```python
from build123d import *

# Parameters (mm, degrees)
BOSS_SWITCH_BODY_DEPTH            = 3
SKETCH1_W                         = 2.994375291
SKETCH1_H                         = 2.409101515
SKETCH1_W_2                       = 3.994375291
SKETCH1_H_2                       = 3.957767538
BOSS_FLANGE_WIDTH_DEPTH           = 5
BOSS_FLANGE_HEIGHT_REACH          = 36.354
SKETCH2_W                         = 4
SKETCH2_H                         = 3.957767538
SKETCH2_W_2                       = 8
SKETCH2_H_2                       = 1.451333978
SKETCH17_W                        = 15.1675
SKETCH17_H                        = 4
BOSS_FLANGE_SUPPORT_DEPTH         = 13.053634428
CUT_WALL_GAP_DEPTH                = 1
TAP_DRILL_FOR_M2X0_4_TAP1_D       = 1.6
M2_CLEARANCE_HOLE2_D              = 2.4
M2_CLEARANCE_HOLE2_DEPTH          = 13.462735941
CHAMFER_FLANGE_SUPPORT_3_SIZE     = 1
FILLET1_R                         = 1
FILLET2_R                         = 0.5
SKETCH28_W                        = 5.9675
SKETCH28_H                        = 12.095866891
CUT_PRINT_SUPPORT_CLEARANCE_DEPTH = 33.624103931


with BuildPart() as part:
    # Sketch-SwitchBossUp → Boss-Switch Body (new body)
    with BuildSketch(Plane.XY):
        with BuildLine():
            Line((-5.697895702, 26.949658376), (-5.524247524, 25.964850623))
            ThreePointArc((-5.524247524, 25.964850623), (-6.169751391, 25.553619307), (-6.3354071, 24.806394693))
            Line((-6.3354071, 24.806394693), (-4.07798079, 12.003893904))
            ThreePointArc((-4.07798079, 12.003893904), (-3.666749473, 11.358390037), (-2.919524859, 11.192734328))
            Line((-2.919524859, 11.192734328), (-2.734924291, 10.145812481))
            Line((-2.734924291, 10.145812481), (-1.956559213, 9.844099378))
            Line((-1.956559213, 9.844099378), (-1.327187553, 9.600139722))
            Line((-1.327187553, 9.600139722), (-1.735258621, 8.547390389))
            ThreePointArc((-1.735258621, 8.547390389), (-1.752158006, 8.457034961), (-1.735258621, 8.366679532))
            Line((-1.735258621, 8.366679532), (-1.327187553, 7.313930199))
            Line((-1.327187553, 7.313930199), (-1.956559213, 7.069970543))
            Line((-1.956559213, 7.069970543), (-0.547014535, 3.433600952))
            Line((-0.547014535, 3.433600952), (0.082357125, 3.677560608))
            Line((0.082357125, 3.677560608), (0.805200549, 1.81275569))
            Line((0.805200549, 1.81275569), (-0.12720191, 1.451333978))
            Line((-0.12720191, 1.451333978), (-0.12720191, 0))
            Line((-0.12720191, 0), (2.867173381, 0))
            Line((2.867173381, 0), (2.867173381, 2.409101515))
            Line((2.867173381, 2.409101515), (2.343664607, 2.409101515))
            Line((2.343664607, 2.409101515), (1.411262148, 2.047679803))
            Line((1.411262148, 2.047679803), (0.688418723, 3.912484721))
            Line((0.688418723, 3.912484721), (1.317790383, 4.156444377))
            Line((1.317790383, 4.156444377), (1.063052687, 4.813621425))
            Line((1.063052687, 4.813621425), (3.125189653, 5.612955517))
            Line((3.125189653, 5.612955517), (3.125189653, 6.948407561))
            Line((3.125189653, 6.948407561), (2.225005405, 7.93492645))
            Line((2.225005405, 7.93492645), (0.162983401, 7.13563692))
            Line((0.162983401, 7.13563692), (-0.091754295, 7.792813968))
            Line((-0.091754295, 7.792813968), (-0.721125955, 7.548854312))
            Line((-0.721125955, 7.548854312), (-1.038134762, 8.366679532))
            ThreePointArc((-1.038134762, 8.366679532), (-1.055034148, 8.457034961), (-1.038134762, 8.547390389))
            Line((-1.038134762, 8.547390389), (-0.721125955, 9.365215609))
            Line((-0.721125955, 9.365215609), (-0.091754295, 9.121255953))
            Line((-0.091754295, 9.121255953), (1.317790383, 12.757625544))
            Line((1.317790383, 12.757625544), (0.688418723, 13.0015852))
            Line((0.688418723, 13.0015852), (1.411262148, 14.866390118))
            Line((1.411262148, 14.866390118), (2.343664607, 14.504968406))
            Line((2.343664607, 14.504968406), (2.867173381, 14.504968406))
            Line((2.867173381, 14.504968406), (2.867173381, 18.462735944))
            Line((2.867173381, 18.462735944), (-0.111637615, 18.462735944))
            Line((-0.111637615, 18.462735944), (-1.12720191, 18.462735944))
            Line((-1.12720191, 18.462735944), (-1.12720191, 15.462735944))
            Line((-1.12720191, 15.462735944), (-0.12720191, 15.462735944))
            Line((-0.12720191, 15.462735944), (0.805200549, 15.101314231))
            Line((0.805200549, 15.101314231), (0.082357125, 13.236509313))
            Line((0.082357125, 13.236509313), (-0.547014535, 13.480468969))
            Line((-0.547014535, 13.480468969), (-1.059112089, 12.159350171))
            Line((-1.059112089, 12.159350171), (-2.346896051, 19.462735944))
            Line((-2.346896051, 19.462735944), (3.767173381, 19.462735944))
            Line((3.767173381, 19.462735944), (3.767173381, 25.857619356))
            Line((3.767173381, 25.857619356), (1.767173381, 25.857619356))
            Line((1.767173381, 25.857619356), (1.767173381, 21.462735944))
            Line((1.767173381, 21.462735944), (-2.699550012, 21.462735944))
            Line((-2.699550012, 21.462735944), (-3.728280196, 27.296954732))
            ThreePointArc((-3.728280196, 27.296954732), (-2.874356585, 27.992742953), (-2.319025652, 28.944012807))
            ThreePointArc((-2.319025652, 28.944012807), (-2.76728001, 29.905297381), (-3.728564583, 29.457043022))
            ThreePointArc((-3.728564583, 29.457043022), (-4.944660137, 28.436617692), (-6.436422172, 28.97957467))
            ThreePointArc((-6.436422172, 28.97957467), (-7.493046212, 29.072017295), (-7.585488837, 28.015393255))
            ThreePointArc((-7.585488837, 28.015393255), (-6.738295005, 27.311426358), (-5.697895702, 26.949658376))
        make_face()
    extrude(amount=BOSS_SWITCH_BODY_DEPTH)

    # Sketch1 → Boss-Flange Width (add)
    with BuildSketch(Plane(origin=(0, 0, 0), x_dir=(-1, 0, 0), z_dir=(0, 0, -1))):
        with Locations((-1.369985736, 1.204550758)):
            Rectangle(SKETCH1_W, SKETCH1_H)
        with Locations((-0.869985736, 16.483852175)):
            Rectangle(SKETCH1_W_2, SKETCH1_H_2)
    extrude(amount=BOSS_FLANGE_WIDTH_DEPTH)

    # Boss-Flange Height: up to this face of the body (flat: up to its plane)
    boss_flange_height_end = Plane(part.part.faces().sort_by_distance((-0.12720191, 1.077409098, -1.438016547))[0])
    # Sketch2 → Boss-Flange Height (add, up to the picked face)
    with BuildSketch(Plane(origin=(-12.300326619, 0, 0), x_dir=(0, 0, -1), z_dir=(1, 0, 0)), mode=Mode.PRIVATE) as boss_flange_height_sk1:
        with Locations((3, 16.483852175)):
            Rectangle(SKETCH2_W, SKETCH2_H)
    boss_flange_height_tool1 = split(extrude(boss_flange_height_sk1.sketch, amount=BOSS_FLANGE_HEIGHT_REACH, mode=Mode.PRIVATE), bisect_by=boss_flange_height_end, keep=Keep.BOTH, mode=Mode.PRIVATE)
    # Sketch2 → Boss-Flange Height (add, up to the picked face)
    with BuildSketch(Plane(origin=(-12.300326619, 0, 0), x_dir=(0, 0, -1), z_dir=(1, 0, 0)), mode=Mode.PRIVATE) as boss_flange_height_sk2:
        with Locations((1, 0.725666989)):
            Rectangle(SKETCH2_W_2, SKETCH2_H_2)
    boss_flange_height_tool2 = split(extrude(boss_flange_height_sk2.sketch, amount=BOSS_FLANGE_HEIGHT_REACH, mode=Mode.PRIVATE), bisect_by=boss_flange_height_end, keep=Keep.BOTH, mode=Mode.PRIVATE)
    add(boss_flange_height_tool1.solids().sort_by(Axis((-12.300327, 16.483852, -3), (1, 0, 0)))[0])
    add(boss_flange_height_tool2.solids().sort_by(Axis((-12.300327, 0.725667, -1), (1, 0, 0)))[0])

    # Sketch17 → Boss-Flange Support (add)
    with BuildSketch(Plane.XZ.offset(-1.451333978)):
        with Locations((-4.716576619, -3)):
            Rectangle(SKETCH17_W, SKETCH17_H)
    extrude(amount=-BOSS_FLANGE_SUPPORT_DEPTH)

    # Sketch27 → Cut-Wall Gap (cut)
    with BuildSketch(Plane.XY):
        Polygon((-0.12720191, 15.462735944), (2.343664607, 14.504968406), (-1.12720191, 14.504968406), (-1.12720191, 15.462735944), align=None)
        Polygon((2.343664607, 2.409101515), (-0.12720191, 2.409101515), (-0.12720191, 1.451333978), align=None)
    extrude(amount=-CUT_WALL_GAP_DEPTH, mode=Mode.SUBTRACT)

    # Tap Drill for M2x0.4 Tap1 (through all)
    with Locations(Plane(origin=(0, 0, 0), x_dir=(-1, 0, 0), z_dir=(0, -1, 0))):
        with Locations((9.300326619, 3), (5.300326619, 3)):
            Hole(TAP_DRILL_FOR_M2X0_4_TAP1_D / 2)

    # M2 Clearance Hole2
    with Locations(Plane.XZ):
        with Locations((-9.300326619, -3), (-5.300326619, -3)):
            Hole(M2_CLEARANCE_HOLE2_D / 2, depth=M2_CLEARANCE_HOLE2_DEPTH)

    # Chamfer-Flange Support 3
    chamfer_flange_support_3_edges = [part.edges().sort_by_distance(p)[0] for p in [
        (-6.213764264, 1.451333978, -1),
    ]]
    chamfer(chamfer_flange_support_3_edges, length=CHAMFER_FLANGE_SUPPORT_3_SIZE)

    # Fillet1
    fillet1_edges = [part.edges().sort_by_distance(p)[0] for p in [
        (-2.734924291, 10.145812481, 1.5),
    ]]
    fillet(fillet1_edges, radius=FILLET1_R)

    # Fillet2
    fillet2_edges = [part.edges().sort_by_distance(p)[0] for p in [
        (-1.956559213, 7.069970543, 1.5),
    ]]
    fillet(fillet2_edges, radius=FILLET2_R)

    # Sketch28 → Cut-Print Support Clearance (cut, through all)
    with BuildSketch(Plane.XY.offset(-1)):
        with Locations((-0.116576619, 8.457034961)):
            Rectangle(SKETCH28_W, SKETCH28_H)
    extrude(amount=-CUT_PRINT_SUPPORT_CLEARANCE_DEPTH, mode=Mode.SUBTRACT)


solid = part.part
```
Verification items for the finished model (mm, model axes). A direction names the side the tool comes from. Give positions to 0.01 mm unless a question says otherwise; leave off trailing zeros. Order: outer loops, then holes, each group sorted by start corner. A loop starts at its lowest first (then second) coordinate and runs counter-clockwise, first axis right, second up. Notation, with made-up numbers: (73, 34) -> (84, 34) arc R21 ccw to (84, 59) -> close; hole circle Ø10 at (51, 23.25). An arc over 180 degrees is marked (long way). One line per item, written item: value.
(1) Draft check along Y on faces 1 (the face through (-10.445, 6.826, -2.64)), 2 (the face through (2.867, 16, -1)), 3 (the face through (-4.92, 28.44, 1.48)). Enter one of: pulls with the +Y half, pulls with the -Y half, needs draft (parallel to the pull), parting line crosses it, or undercut.
Final values:
face 1: needs draft
face 2: undercut
face 3: pulls with the +Y half
(2) Gauge pin test, flat ends, axial feed: pin 1 (0.6 mm diameter, centred on x = 2.5, z = 1.5, fed in from +Y); pin 2 (2 mm diameter, centred on x = -5.3, z = -3, fed in from +Y); pin 3 (3.5 mm diameter, centred on y = 17, z = 0.5, fed in from -X); pin 4 (3 mm diameter, centred on x = -1, z = -1, fed in from +Y). Record the tip position at first contact, or that the pin passes through.
Final values:
pin 1: y = 25.86
pin 2: y = 18.46
pin 3: x = -12.3
pin 4: y = 21.46
(3) Sectioned sample at B-B on x = -9. Record the cut outline in (y, z), then the cut area to 3 significant figures.
Final values:
outline: (0, -5) -> (18.46, -5) -> (18.46, -3.74) -> (13.46, -3.74) -> (13.46, -4.16) -> (0, -4.16) -> close; (0, -1.84) -> (13.46, -1.84) -> (13.46, -2.26) -> (18.46, -2.26) -> (18.46, -1) -> (2.45, -1) -> (1.45, 0) -> (1.45, 3) -> (0, 3) -> close
area: 41.5 mm^2
(4) Sectioned sample at A-A on z = -3. Record the cut outline in (x, y).
Final values:
outline: (-12.3, 0) -> (-10.5, 0) -> (-10.5, 13.46) -> (-10.1, 13.46) -> (-10.1, 18.46) -> (-12.3, 18.46) -> close; (-8.5, 13.46) -> (-8.1, 13.46) -> (-8.1, 0) -> (-6.5, 0) -> (-6.5, 13.46) -> (-6.1, 13.46) -> (-6.1, 18.46) -> (-8.5, 18.46) -> close; (-4.5, 13.46) -> (-4.1, 13.46) -> (-4.1, 0) -> (2.87, 0) -> (2.87, 2.41) -> (-3.1, 2.41) -> (-3.1, 14.5) -> (2.87, 14.5) -> (2.87, 18.46) -> (-4.5, 18.46) -> close
(5) Scan lines: line 1 along X through (y, z) = (14.95, -3); line 2 along Z through (x, y) = (-3.25, 16.5); line 3 along Y through (x, z) = (-8.75, 2.75). Record each from-to range of solid material in increasing order. Write a range as [from, to].
Final values:
line 1: [-12.3, -10.1], [-8.5, -6.1], [-4.5, 2.87]
line 2: [-5, -1], [0, 3]
line 3: [0, 1.45]
(6) Tool access check on faces 4 (the face through (-1.17, 5.04, 1.48)), 5 (the face through (1.767, 24, 1)), 6 (the face through (1.045, 13.921, 1.479)), 7 (the face through (1.21, 7.54, 1.48)), 8 (the face through (-2.5, 18, 0)). Record the directions out of +Z, -Z, +X, -X, +Y, -Y that give a thin tool (end or side, any length) a straight path to the whole face; none if there is none.
Final values:
face 4: +Z, -Z, -X
face 5: +Z, -Z, +Y
face 6: +Z
face 7: +Z, -Z
face 8: -X
